Work out the finished part from the listing and answer in its coordinate system (mm). Coordinates: 2 decimals unless noted, no trailing zeros. Order: outer loops, then holes, each group sorted by start corner. A loop starts at its lowest first (then second) coordinate and runs counter-clockwise, first axis right, second up.
1. Determine the mould class of faces 1 (the cylindrical face through (-59.6, 9.66, -58.38)), 2 (the cylindrical face through (67.278, 9.658, 58.716)), 3 (the flat face through (73.025, 9, 1)), 4 (the flat face through (1, 9, -101.6)) for opening direction X: +X half, -X half, draft (parallel to the pull), parting line (faces both ways), or undercut.
2. The part is cut by section B-B, the plane z = 57.15. Give the vertices of the cut face in (x, y) (3 decimals), then the cut area to 3 significant figures.
3. The part is cut by section A-A, the plane x = -63.5. Give the vertices of the cut face in (y, z).
4. Find the intervals of material crossed by probe 1 along X at (y, z) = (11.75, 57.15) (3 decimals); probe 2 along Z at (x, y) = (63.5, 6.75); probe 3 along X at (y, z) = (1, 54) (3 decimals), in increasing order.
Autodesk Inventor part; units mm, degrees
ref_plane "YZ Plane" through (0, 0, 0) normal (1, 0, 0) x (0, 1, 0)
ref_plane "XZ Plane" through (0, 0, 0) normal (0, 1, 0) x (-1, 0, 0)
ref_plane "XY Plane" through (0, 0, 0) normal (0, 0, 1) x (1, 0, 0)
sketch "Sketch1" plane through (0, 0, 0) normal (0, 1, 0) x (-1, 0, 0)
  line L0 (73.025, 101.6) -> (-73.025, 101.6)
  line L1 (-73.025, 101.6) -> (-73.025, -101.6)
  line L2 (-73.025, -101.6) -> (73.025, -101.6)
  line L3 (73.025, -101.6) -> (73.025, 101.6)
  line L4 (73.025, 101.6) -> (-73.025, -101.6) construction
  line L5 (-73.025, 101.6) -> (73.025, -101.6) construction
  point P0 (0, 0)
  dimension "d0" = 146.05
  dimension "d1" = 203.2
extrude "Extrusion1" add sketch "Sketch1" along normal blind 19.05
sketch "Sketch2" plane through (0, 19.05, 0) normal (0, 1, 0) x (1, 0, 0)
  circle A0 centre (-63.5, -57.15) radius 4.0894
  circle A1 centre (-63.5, 0) radius 4.0894
  circle A2 centre (-63.5, 57.15) radius 4.0894
  circle A3 centre (63.5, -57.15) radius 4.0894
  circle A4 centre (63.5, 0) radius 4.0894
  circle A5 centre (63.5, 57.15) radius 4.0894
  line L0 (-73.025, -101.6) -> (73.025, -101.6)
  line L1 (73.025, -101.6) -> (73.025, 101.6)
  line L2 (-73.025, 101.6) -> (-73.025, -101.6)
  point P0 (0, 0)
  dimension "d4" = 8.1788
  dimension "d5" = 8.1788
  dimension "d6" = 8.1788
  dimension "d7" = 8.1788
  dimension "d8" = 8.1788
  dimension "d9" = 8.1788
  dimension "d10" = 44.45
  dimension "d11" = 101.6
  dimension "d12" = 158.75
  dimension "d13" = 44.45
  dimension "d14" = 101.6
  dimension "d15" = 158.75
  dimension "d16" = 9.525
  dimension "d17" = 9.525
  dimension "d18" = 9.525
  dimension "d19" = 9.525
  dimension "d20" = 9.525
  dimension "d21" = 9.525
extrude "Extrusion2" cut sketch "Sketch2" against normal blind 19.05
properties part number "Part_Back"
Geometry says:
1. face 1: undercut
1. face 2: undercut
1. face 3: +X half
1. face 4: draft
2. outline: (-73.025, 0) - (-67.589, 0) - (-67.589, 19.05) - (-73.025, 19.05) - close; (-59.411, 0) - (59.411, 0) - (59.411, 19.05) - (-59.411, 19.05) - close; (67.589, 0) - (73.025, 0) - (73.025, 19.05) - (67.589, 19.05) - close
2. area: 2,470 mm2
3. outline: (0, -101.6) - (19.05, -101.6) - (19.05, -61.24) - (0, -61.24) - close; (0, -53.06) - (19.05, -53.06) - (19.05, -4.09) - (0, -4.09) - close; (0, 4.09) - (19.05, 4.09) - (19.05, 53.06) - (0, 53.06) - close; (0, 61.24) - (19.05, 61.24) - (19.05, 101.6) - (0, 101.6) - close
4. probe 1: x = -73.025 to -67.589, -59.411 to 59.411, 67.589 to 73.025
4. probe 2: z = -101.6 to -61.24, -53.06 to -4.09, 4.09 to 53.06, 61.24 to 101.6
4. probe 3: x = -73.025 to -66.108, -60.892 to 60.892, 66.108 to 73.025
